from build123d import *

# Parameters (mm, degrees)
BOSS_EXTRUDE1_DEPTH = 40
SKETCH2_R           = 4
CUT_EXTRUDE1_DEPTH  = 40
SKETCH3_R           = 4
CUT_EXTRUDE2_DEPTH  = 40
BOSS_EXTRUDE4_DEPTH = 18
BOSS_EXTRUDE5_REACH = 69.506
RIB7_REACH          = 62.042
SKETCH14_WALL_W     = 149.669532934
SKETCH14_WALL_H     = 6
CUT_EXTRUDE7_DEPTH  = 30
CUT_EXTRUDE8_START  = 30
SKETCH18_R          = 18
SKETCH18_R_2        = 15
CUT_EXTRUDE8_DEPTH  = 30
SKETCH16_R          = 18
SKETCH16_R_2        = 15
CUT_EXTRUDE5_DEPTH  = 18


with BuildPart() as part:
    # Sketch1 → Boss-Extrude1 (new body)
    with BuildSketch(Plane.XY):
        with BuildLine():
            Line((0, 0), (9, 0))
            Line((9, 0), (9, -14))
            Line((9, -14), (46, -14))
            Line((46, -14), (46, -5))
            Line((46, -5), (17, -5))
            ThreePointArc((17, -5), (15.585786438, -4.414213562), (15, -3))
            Line((15, -3), (15, 7))
            ThreePointArc((15, 7), (14.414213562, 8.414213562), (13, 9))
            Line((13, 9), (0, 9))
            Line((0, 9), (0, 0))
        make_face()
    extrude(amount=-BOSS_EXTRUDE1_DEPTH)

    # Sketch2 → Cut-Extrude1 (cut)
    with BuildSketch(Plane(origin=(0, -5, 0), x_dir=(1, 0, 0), z_dir=(0, 1, 0))):
        with Locations(Location((36, 9, 0), (0, 0, 180))):
            Circle(SKETCH2_R)
    extrude(amount=-CUT_EXTRUDE1_DEPTH, mode=Mode.SUBTRACT)

    # Sketch3 → Cut-Extrude2 (cut)
    with BuildSketch(Plane(origin=(0, -5, 0), x_dir=(1, 0, 0), z_dir=(0, 1, 0))):
        with Locations(Location((36, 31, 0), (0, 0, 180))):
            Circle(SKETCH3_R)
    extrude(amount=-CUT_EXTRUDE2_DEPTH, mode=Mode.SUBTRACT)

    # Sketch7 → Boss-Extrude5 (add, up to next)
    with BuildSketch(Plane(origin=(0, 15, 0), x_dir=(1, 0, 0), z_dir=(0, 1, 0)), mode=Mode.PRIVATE) as boss_extrude5_sk1:
        with BuildLine():
            Line((0, 2), (0, 20))
            Line((0, 20), (0, 38))
            ThreePointArc((0, 38), (18, 20), (0, 2))
        make_face()
    boss_extrude5_tool1 = extrude(boss_extrude5_sk1.sketch, amount=-BOSS_EXTRUDE5_REACH, mode=Mode.PRIVATE) - part.part


with BuildPart() as body_2:
    # Sketch4 → Boss-Extrude4 (new body)
    with BuildSketch(Plane(origin=(0, 15, 0), x_dir=(1, 0, 0), z_dir=(0, 1, 0))):
        with BuildLine():
            Line((0, 30), (0, 35))
            ThreePointArc((0, 35), (15, 20), (0, 5))
            Line((0, 5), (0, 10))
            ThreePointArc((0, 10), (10, 20), (0, 30))
        make_face()
    extrude(amount=BOSS_EXTRUDE4_DEPTH)


with BuildPart() as part_1:
    add(part.part)

    add(body_2.part)  # Boss-Extrude5 merges body 2
    add(boss_extrude5_tool1.solids().sort_by_distance((7.639437, 15, -20))[0])

    # Sketch14 wall → Rib7 (add, up to next)
    with BuildSketch(Plane(origin=(27.5, 5, -20), x_dir=(-0.688749461915, 0.724999433594, 0), z_dir=(0.724999433594, 0.688749461915, 0)), mode=Mode.PRIVATE) as rib7_sk1:
        Rectangle(SKETCH14_WALL_W, SKETCH14_WALL_H)
    rib7_tool1 = extrude(rib7_sk1.sketch, amount=-RIB7_REACH, mode=Mode.PRIVATE) - part_1.part
    add(rib7_tool1.solids().sort_by_distance((27.5, 5, -20))[0])

    # Sketch17 → Cut-Extrude7 (cut)
    with BuildSketch(Plane(origin=(46, 0, 0), x_dir=(0, 0, -1), z_dir=(1, 0, 0))):
        Polygon((20, 15), (35.006710278, 15), (35.006710278, 24.792153867), (20, 24.792153867), (5.167377758, 24.792153867), (5.167377758, 15), align=None)
    extrude(amount=-CUT_EXTRUDE7_DEPTH, mode=Mode.SUBTRACT)

    # Sketch18 → Cut-Extrude8 (cut)
    with BuildSketch(Plane(origin=(0, 15, 0), x_dir=(1, 0, 0), z_dir=(0, 1, 0)).offset(CUT_EXTRUDE8_START)):
        with Locations((0, 20)):
            Circle(SKETCH18_R)
        with Locations((0, 20)):
            Circle(SKETCH18_R_2, mode=Mode.SUBTRACT)
    extrude(amount=-CUT_EXTRUDE8_DEPTH, mode=Mode.SUBTRACT)

    # Mirror13: part across plane


with BuildPart() as part_2:
    add(part_1.part)
    add(part_1.part.mirror(Plane(origin=(0, 0, -40), x_dir=(0, 0, 1), z_dir=(-1, 0, 0))))

    # Sketch16 → Cut-Extrude5 (cut)
    with BuildSketch(Plane(origin=(0, 15, 0), x_dir=(1, 0, 0), z_dir=(0, 1, 0))):
        with Locations((0, 20)):
            Circle(SKETCH16_R)
        with Locations(Location((0, 20, 0), (0, 0, 180))):
            Circle(SKETCH16_R_2, mode=Mode.SUBTRACT)
    extrude(amount=CUT_EXTRUDE5_DEPTH, mode=Mode.SUBTRACT)


solid = part_2.part
Check sheet for the modelled part. Datum: model origin and axes. Units: mm. A direction names the side the tool comes from. Coordinates: 2 decimals unless noted, no trailing zeros. Write each loop counter-clockwise with the first axis right and the second up, starting at its lowest first coordinate (ties: lowest second). Pieces come first, ordered by that corner, then holes.
Item 1: Scan lines: probe 1 along Z at (x, y) = (36, -10); probe 2 along Z at (x, y) = (0, 24); probe 3 along X at (y, z) = (-11, -36). Record each from-to range of solid material in increasing order.
Numbers:
probe 1: z = -40 to -35, -27 to -13, -5 to 0
probe 2: z = -35 to -30, -10 to -5
probe 3: x = -46 to -9, 9 to 46
Item 2: Cross-section at B-B on z = -31. Count the separate pieces of the cut face and the enclosed holes in it, then the cut area to 3 significant figures.
Numbers:
separate pieces: 3
enclosed holes: 0
area: 1,390 mm2
Item 3: Mould release check, pull along X, two halves, no side actions. Record for faces 1 (the face through (-15, 2, -5)), 2 (the face through (-9, -7, -20)), 3 (the face through (24, 1, -17)): released by +X, released by -X, zero draft, split by the parting line, or undercut.
Numbers:
face 1: released by -X
face 2: undercut
face 3: zero draft
Item 4: Cross-section at A-A on y = -11. Record the boundary of the cut face in (x, z).
Numbers:
outline: (-46, -40) - (-9, -40) - (-9, 0) - (-46, 0) - close; (9, -40) - (46, -40) - (46, 0) - (9, 0) - close; hole circle Ø8 at (-36, -31); hole circle Ø8 at (-36, -9); hole circle Ø8 at (36, -31); hole circle Ø8 at (36, -9)
Item 5: Cross-section at D-D on y = 25.5. Record the boundary of the cut face in (x, z), then the cut area to 3 significant figures.
Numbers:
outline: circle Ø30 at (0, -20); hole circle Ø20 at (0, -20)
area: 393 mm2
Item 6: Access from +Z, -Z, +X, -X, +Y, -Y to the whole of each face (thin tool, end or side, straight path). Record for faces 4 (the face through (0, 10, -38)), 5 (the face through (-14.43, 8.4, -4.95)), 6 (the face through (-15, 2, -35)).
Numbers:
face 4: -Z, +Y
face 5: +Z, -X, +Y
face 6: -Z, -X, +Y
Item 7: Depth check by flat-ended pin: pin 1 Ø16 at (x, z) = (0, -20) entering from +Y; pin 2 Ø3 at (y, z) = (1, -6.5) entering from +X; pin 3 Ø8 at (y, z) = (0.5, -34) entering from -X; pin 4 Ø6 at (x, y) = (-29.5, 7.5) entering from +Z. Enter the tip coordinate at first touch or a pass-through.
Numbers:
pin 1: stops at y = 15
pin 2: stops at x = 15
pin 3: stops at x = -15.06
pin 4: passes through
Item 8: Cross-section at C-C on x = -36. Record the boundary of the cut face in (y, z), then the cut area to 3 significant figures.
Numbers:
outline: (-14, -40) - (-5, -40) - (-5, -35) - (-14, -35) - close; (-14, -27) - (-5, -27) - (-5, -23) - (-3.95, -23) - (-3.95, -17) - (-5, -17) - (-5, -13) - (-14, -13) - close; (-14, -5) - (-5, -5) - (-5, 0) - (-14, 0) - close
area: 222 mm2
